Autodesk Inventor part; units mm, degrees
ref_plane "Work Plane1" through (-12.4, 3, 56.4645) normal (0, 0, 1) x (0, 1, 0)
ref_plane "YZ Plane" through (0, 0, 0) normal (1, 0, 0) x (0, 1, 0)
ref_plane "XZ Plane" through (0, 0, 0) normal (0, 1, 0) x (-1, 0, 0)
sketch "Sketch1" plane through (0, 0, 0) normal (0, 1, 0) x (-1, 0, 0)
  line L0 (12.4, 56.4645) -> (22.5, 56.4645) construction
  circle A0 centre (0, 0) radius 1.5
  line L1 (12.4, 56.4645) -> (0, 0) construction
  circle A1 centre (60, 0) radius 1.5
  line L2 (0, 0) -> (60, 0) construction
  line L3 (47.6, 56.4645) -> (37.5, 56.4645) construction
  line L4 (60, 0) -> (47.6, 56.4645) construction
  line L5 (47.6, 56.4645) -> (37.5, 56.4645) construction
  line L6 (36, 58.4645) -> (24, 58.4645) construction
  line L7 (37.5, 56.4645) -> (36, 58.4645) construction
  line L8 (36, 58.4645) -> (24, 58.4645) construction
  line L9 (24, 58.4645) -> (22.5, 56.4645) construction
  line L10 (22.5, 56.4645) -> (12.4, 56.4645) construction
  line L11 (47.6, 56.4645) -> (47.6, 59.4645)
  line L12 (47.6, 59.4645) -> (37.5, 59.4645)
  line L13 (37.5, 59.4645) -> (37.5, 56.4645)
  line L14 (37.5, 56.4645) -> (22.5, 56.4645)
  line L15 (22.5, 56.4645) -> (22.5, 59.4645)
  line L16 (22.5, 59.4645) -> (12.4, 59.4645)
  line L17 (12.4, 59.4645) -> (12.4, 56.4645)
  circle A2 centre (60, 0) radius 5
  circle A3 centre (0, 0) radius 5
  line L18 (47.6, 56.4645) -> (64.7726, 1.4908)
  line L19 (12.4, 56.4645) -> (-4.7726, 1.4908)
  line L20 (0, -5) -> (60, -5)
  point P0 (17, 90.5)
  dimension "d0" = 3
  dimension "d1" = 10.1
  dimension "d2" = 3
  dimension "d3" = 10.1
  dimension "d4" = 10
  dimension "d5" = 10
  dimension "d6" = 3
  dimension "d7" = 3
extrude "Extrusion1" add sketch "Sketch1" along normal blind 3
sketch "Sketch2" plane through (0, 3, 0) normal (0, 1, 0) x (1, 0, 0)
  line L0 (-47.6, -56.4645) -> (-47.6, -59.4645)
  line L1 (-37.5, -59.4645) -> (-37.5, -56.4645)
  line L2 (-47.6, -59.4645) -> (-37.5, -59.4645)
  line L3 (-37.5, -59.4645) -> (-37.5, -56.4645)
  line L4 (-37.5, -56.4645) -> (-47.6, -56.4645)
  line L5 (-47.6, -56.4645) -> (-47.6, -59.4645)
  line L6 (-12.4, -59.4645) -> (-12.4, -56.4645)
  line L7 (-37.5, -56.4645) -> (-22.5, -56.4645)
  line L8 (-12.4, -59.4645) -> (-22.5, -59.4645)
  line L9 (-22.5, -59.4645) -> (-22.5, -56.4645)
  line L10 (-22.5, -56.4645) -> (-12.4, -56.4645)
  line L11 (-12.4, -56.4645) -> (-12.4, -59.4645)
  point P0 (0, 0)
extrude "Extrusion2" add sketch "Sketch2" along normal blind 4.6
ref_plane "Work Plane1" through (-12.4, 3, 56.4645) normal (0, 0, 1) x (0, 1, 0)
sketch "Sketch3" plane through (-12.4, 3, 56.4645) normal (0, 0, 1) x (0, 1, 0)
  line L0 (0, 0) -> (4.6, 0)
  line L1 (-3, 10.1) -> (4.6, 10.1)
  line L2 (4.6, 0) -> (1.6, 0)
  line L3 (1.6, 0) -> (1.6, 10.1)
  line L4 (1.6, 10.1) -> (4.6, 10.1)
  line L5 (4.6, 10.1) -> (4.6, 0)
  line L6 (-3, 25.1) -> (4.6, 25.1)
  line L7 (-3, 35.2) -> (4.6, 35.2)
  line L8 (4.6, 25.1) -> (1.6, 25.1)
  line L9 (1.6, 25.1) -> (1.6, 35.2)
  line L10 (1.6, 35.2) -> (4.6, 35.2)
  line L11 (4.6, 35.2) -> (4.6, 25.1)
  point P0 (-3, -12.4)
  point P1 (1.6, 25.1)
  dimension "d12" = 3
  dimension "d13" = 3
extrude "Extrusion3" add sketch "Sketch3" against normal blind 3
fillet "Fillet1" radius 2 4 edges at (-12.4, 6.1, 53.4645) (-22.5, 6.1, 53.4645) (-37.5, 6.1, 53.4645) (-47.6, 6.1, 53.4645)
sketch "Sketch4" plane through (0, 3, 0) normal (0, 1, 0) x (1, 0, 0)
  circle A0 centre (-10, -5) radius 4.5
  line L0 (0, 5) -> (-60, 5)
  circle A1 centre (0, 0) radius 1.5 construction
  line L1 (0, 0) -> (0, -9.5) construction
  circle A2 centre (-50, -5) radius 4.5
  circle A3 centre (-10, -45) radius 4.5
  circle A4 centre (-50, -45) radius 4.5
  circle A5 centre (-10, -5) radius 0.5
  circle A6 centre (-50, -5) radius 0.5
  circle A7 centre (-50, -45) radius 0.5
  circle A8 centre (-10, -45) radius 0.5
  dimension "d18" = 9
  dimension "d27" = 60
  dimension "d28" = 10
  dimension "d29" = 10
  dimension "d32" = 40
  dimension "d35" = 40
  dimension "d53" = 1
  dimension "d54" = 1
  dimension "d55" = 1
  dimension "d56" = 1
extrude "Extrusion4" add sketch "Sketch4" against normal blind 3 contours A0 | A2 | A3 | A4 | A5 | A6 | A7 | A8
sketch "Sketch6" plane through (0, 0, 0) normal (0, -1, 0) x (1, 0, 0)
  circle A0 centre (-60, 0) radius 1.55 construction
  line L0 (-44.1169, 11.8645) -> (-48.1306, 17.0674)
  line L1 (-60, 0) -> (-44.1169, 11.8645) construction
  line L2 (-44.1169, 11.8645) -> (-48.1306, 17.0674)
  line L3 (-48.1306, 17.0674) -> (-40.0449, 32.3645)
  line L4 (-48.1306, 17.0674) -> (-40.0449, 32.3645)
  line L5 (-40.0449, 32.3645) -> (-35.7189, 32.3645)
  line L6 (-40.0449, 32.3645) -> (-35.7189, 32.3645)
  line L7 (-33.9689, 33.3645) -> (-26.0311, 33.3645)
  line L8 (-35.7189, 32.3645) -> (-33.9689, 33.3645)
  line L9 (-33.9689, 33.3645) -> (-26.0311, 33.3645)
  line L10 (-24.2811, 32.3645) -> (-19.9551, 32.3645)
  line L11 (-26.0311, 33.3645) -> (-24.2811, 32.3645)
  line L12 (-24.2811, 32.3645) -> (-19.9551, 32.3645)
  line L13 (-19.9551, 32.3645) -> (-11.8694, 17.0674)
  line L14 (-11.8694, 17.0674) -> (-15.9122, 11.8645)
  line L15 (-15.8831, 11.8645) -> (-19.4, 11.8645)
  line L16 (-15.9122, 11.8645) -> (-19.4, 11.8645)
  line L17 (-19.4, 11.8645) -> (-20.9, 13.8645)
  line L18 (-19.4, 11.8645) -> (-20.9, 13.8645)
  line L19 (-20.9, 13.8645) -> (-39.1, 13.8645)
  line L20 (-20.9, 13.8645) -> (-39.1, 13.8645)
  line L21 (-39.1, 13.8645) -> (-40.6, 11.8645)
  line L22 (-39.1, 13.8645) -> (-40.6, 11.8645)
  line L23 (-40.6, 11.8645) -> (-44.1169, 11.8645)
  line L24 (-40.6, 11.8645) -> (-44.1169, 11.8645)
  circle A1 centre (-60, 0) radius 1.5 construction
  point P0 (0, 0)
  point P1 (17, 90.5)
extrude "Extrusion6" cut sketch "Sketch6" against normal up to next
extrude "Extrusion8" cut sketch "Sketch4" against normal up to next contours A5 | A6 | A7 | A8
properties part number "ElectronicsMount - ClipOnStyle"
Geometry check sheet. Reference: the model listing, model coordinates, mm. A direction names the side the tool comes from. Round coordinates to 2 decimals unless told otherwise and drop trailing zeros. Order: outer loops, then holes, each group sorted by start corner. A loop starts at its lowest first (then second) coordinate and runs counter-clockwise, first axis right, second up. Notation, with made-up numbers: (-38.75, -16.75) -> (-24.75, -16.75) arc R19 cw to (-24.75, 9.25) -> close; hole circle Ø6 at (-27.75, 2.5). An arc over 180 degrees is marked (long way). Return JSON: item names as keys, results as strings. Group by question number.
Q1. Material ranges on probe 1 along Z at (x, y) = (-50, 1.4); probe 2 along X at (y, z) = (1, 5); probe 3 along Y at (x, z) = (-46.5, 14), recorded low to high. Write a range as from..to.
Q2. Section check D-D, the plane z = 9. Record the boundary of the cut face in (x, y), plus the area to 3 significant figures.
Q3. Gauge pin test, flat ends, axial feed: pin 1 (4.5 mm diameter, centred on y = 5.5, z = 58, fed in from -X); pin 2 (1.5 mm diameter, centred on x = -33.5, y = 2, fed in from +Z); pin 3 (4.5 mm diameter, centred on y = 3, z = 57.5, fed in from +X); pin 4 (2 mm diameter, centred on y = 4.5, z = 33, fed in from -X). Record the tip position at first contact, or that the pin passes through.
Q4. Tool access check on faces 5 (the flat face through (-30, 1, 56.464)), 6 (the flat face through (-46.096, 1.479, 14.43)), 7 (the cylindrical face through (-12.97, 6.121, 54.066)). Record the directions out of +Z, -Z, +X, -X, +Y, -Y that give a thin tool (end or side, any length) a straight path to the whole face; none if there is none.
Q5. Release check for a two-part mould opening along X. For faces 1 (the cylindrical face through (-46.999, 6.121, 54.035)), 2 (the flat face through (-30, 3, 13)), 3 (the flat face through (-42, 1, 11.864)), 4 (the flat face through (-22, 1, 32.364)) record: released by +X, released by -X, zero draft, split by the parting line, or undercut.
Q6. Section check C-C, the plane y = 1.5. Count the separate pieces of the cut face and the enclosed holes in it, plus the area to 3 significant figures.
Q7. Section check B-B, the plane z = 0. Record the boundary of the cut face in (x, y), plus the area to 3 significant figures.
Q8. Section check A-A, the plane y = 6.25. Record the boundary of the cut face in (x, z), plus the area to 3 significant figures.
Numbers:
{
 "1": {"probe 1": "-5..4.5, 5.5..44.5, 45.5..49.5", "probe 2": "-63.68..-50.5, -49.5..-10.5, -9.5..3.68", "probe 3": "0..3"},
 "2": {"outline": "(-62.43, 0) -> (2.43, 0) -> (2.43, 3) -> (-62.43, 3) -> close", "area": "195 mm^2"},
 "3": {"pin 1": "x = -47.6", "pin 2": "z = 56.46", "pin 3": "x = -12.02", "pin 4": "through"},
 "4": {"face 5": "+Z, +Y, -Y", "face 6": "+Y, -Y", "face 7": "-Z, +X, +Y"},
 "5": {"face 1": "released by -X", "face 2": "zero draft", "face 3": "undercut", "face 4": "undercut"},
 "6": {"separate pieces": "1", "enclosed holes": "7", "area": "2,840 mm^2"},
 "7": {"outline": "(-65, 0) -> (-61.5, 0) -> (-61.5, 3) -> (-65, 3) -> close; (-58.5, 0) -> (-1.5, 0) -> (-1.5, 3) -> (-58.5, 3) -> close; (1.5, 0) -> (5, 0) -> (5, 3) -> (1.5, 3) -> close", "area": "192 mm^2"},
 "8": {"outline": "(-47.6, 55.46) arc R2 ccw to (-45.6, 53.46) -> (-39.5, 53.46) arc R2 ccw to (-37.5, 55.46) -> (-37.5, 59.46) -> (-47.6, 59.46) -> close; (-22.5, 55.46) arc R2 ccw to (-20.5, 53.46) -> (-14.4, 53.46) arc R2 ccw to (-12.4, 55.46) -> (-12.4, 59.46) -> (-22.5, 59.46) -> close", "area": "118 mm^2"}
}
